from build123d import *

# Parameters (mm, degrees)
BOSS_EXTRUDE1_DEPTH = 80
CUT_EXTRUDE4_DEPTH  = 86.022442091
SKETCH3_W           = 85.02244209
SKETCH3_H           = 14.481412897
CUT_EXTRUDE5_DEPTH  = 61.793248749
SKETCH4_R           = 11.893880873
CUT_EXTRUDE6_DEPTH  = 86.022442091


with BuildPart() as part:
    # Sketch1 → Boss-Extrude1 (new body)
    with BuildSketch(Plane.XY):
        with BuildLine():
            Line((40.088301711, 44.273344197), (40.088301711, -18.282027703))
            ThreePointArc((40.088301711, -18.282027703), (-2.422919334, -60.793248749), (-44.934140379, -18.282027703))
            Line((-44.934140379, -18.282027703), (-44.934140379, 44.273344197))
            Line((-44.934140379, 44.273344197), (-28.193970434, 44.273344197))
            Line((-28.193970434, 44.273344197), (-28.193970434, -18.282027703))
            ThreePointArc((-28.193970434, -18.282027703), (-2.643184728, -43.832813409), (22.907600978, -18.282027703))
            Line((22.907600978, -18.282027703), (22.907600978, 44.273344197))
            Line((22.907600978, 44.273344197), (40.088301711, 44.273344197))
        make_face()
    extrude(amount=-BOSS_EXTRUDE1_DEPTH)

    # Sketch2 → Cut-Extrude4 (cut, through all)
    with BuildSketch(Plane(origin=(40.088301711, 0, 0), x_dir=(0, 0, -1), z_dir=(1, 0, 0))):
        with BuildLine():
            Line((14.481412897, -18.282027703), (14.481412897, 12.995658247))
            ThreePointArc((14.481412897, 12.995658247), (40, 38.51424535), (65.518587103, 12.995658247))
            Line((65.518587103, 12.995658247), (65.518587103, -18.282027703))
            Line((65.518587103, -18.282027703), (80, -18.282027703))
            Line((80, -18.282027703), (80, 44.273344197))
            Line((80, 44.273344197), (0, 44.273344197))
            Line((0, 44.273344197), (0, -18.282027703))
            Line((0, -18.282027703), (14.481412897, -18.282027703))
        make_face()
    extrude(amount=-CUT_EXTRUDE4_DEPTH, mode=Mode.SUBTRACT)

    # Sketch3 → Cut-Extrude5 (cut, through all)
    with BuildSketch(Plane(origin=(0, 0, 0), x_dir=(1, 0, 0), z_dir=(0, 1, 0))):
        with Locations((-2.422919334, 7.240706449)):
            Rectangle(SKETCH3_W, SKETCH3_H)
        with Locations((-2.422919334, 72.759293552)):
            Rectangle(SKETCH3_W, SKETCH3_H)
    extrude(amount=-CUT_EXTRUDE5_DEPTH, mode=Mode.SUBTRACT)

    # Sketch4 → Cut-Extrude6 (cut, through all)
    with BuildSketch(Plane(origin=(40.088301711, 0, 0), x_dir=(0, 0, -1), z_dir=(1, 0, 0))):
        with Locations((40, 12.995658247)):
            Circle(SKETCH4_R)
    extrude(amount=-CUT_EXTRUDE6_DEPTH, mode=Mode.SUBTRACT)


solid = part.part
Check sheet for the modelled part. Datum: model origin and axes. Units: mm. A direction names the side the tool comes from. Give positions to 0.01 mm unless a question says otherwise; leave off trailing zeros. Loops run counter-clockwise (first coordinate to the right, second up) from the corner with the lowest first, then second, coordinate; pieces in that order, holes last. Notation, with made-up numbers: M 15,25.5 L 62,25.5 A5 cw 62,33.5 Z; hole C 8,22 d9. An arc over 180 degrees is marked long. Use a Markdown table: item, result. Add a question column.
Q1. Go/stop test with flat-tipped pins: pin 1 (3 mm diameter, centred on x = -20.5, z = -43, fed in from +Y); pin 2 (10 mm diameter, centred on x = 27.5, z = -55.5, fed in from -Y); pin 3 (1.5 mm diameter, centred on x = -34.5, z = -34, fed in from +Y). Record where each tip stops, or that it passes through.
Q2. Sectioned sample at A-A, the plane y = -14.5. Record the cut outline in (x, z), then the cut area to 3 significant figures.
Q3. Sectioned sample at C-C, the plane y = -41. Record the cut outline in (x, z), then the cut area to 3 significant figures.
Q4. Scan lines: line 1 along X through (y, z) = (-11, -56); line 2 along X through (y, z) = (-22, -52); line 3 along Y through (x, z) = (26, -31). Record each from-to range of solid material in increasing order. Write a range as [from, to].
Q5. Sectioned sample at D-D, the plane z = -24. Record the cut outline in (x, y).
Q6. Mould release check, pull along X, two halves, no side actions. Record for faces 1 (the flat face through (-3, -48, -65.519)), 2 (the cylindrical face through (-3.205, -43.827, -39.643)), 3 (the cylindrical face through (-1.488, -60.783, -39.643)), 4 (the flat face through (-44.934, -3, -40)): pulls with the +X half, pulls with the -X half, needs draft (parallel to the pull), parting line crosses it, or undercut.
Q7. Sectioned sample at B-B, the plane z = -40. Record the cut outline in (x, y).
Q8. Tool access check on faces 5 (the flat face through (22.908, -3, -40)), 6 (the cylindrical face through (-36.45, 38.51, -39.44)). Record the directions out of +Z, -Z, +X, -X, +Y, -Y that give a thin tool (end or side, any length) a straight path to the whole face; none if there is none.
Verdict:
| question | item | result |
|---|---|---|
| 1 | pin 1 | y = -34.96 |
| 1 | pin 2 | y = -52.72 |
| 1 | pin 3 | y = 37.97 |
| 2 | outline | M -44.93,-65.52 L -28.19,-65.52 L -28.19,-14.48 L -44.93,-14.48 Z; M 22.91,-65.52 L 40.09,-65.52 L 40.09,-14.48 L 22.91,-14.48 Z |
| 2 | area | 1,730 mm^2 |
| 3 | outline | M -38.35,-65.52 L -14.34,-65.52 L -14.34,-14.48 L -38.35,-14.48 Z; M 9.05,-65.52 L 33.51,-65.52 L 33.51,-14.48 L 9.05,-14.48 Z |
| 3 | area | 2,470 mm^2 |
| 4 | line 1 | [-44.93, -28.19], [22.91, 40.09] |
| 4 | line 2 | [-44.77, -27.92], [22.64, 39.93] |
| 4 | line 3 | [-49.89, 5.22], [20.77, 36.87] |
| 5 | outline | M -44.93,-18.28 A42.51 ccw 40.09,-18.28 L 40.09,32.88 L 22.91,32.88 L 22.91,-18.28 A25.55 cw -28.19,-18.28 L -28.19,32.88 L -44.93,32.88 Z |
| 6 | face 1 | needs draft |
| 6 | face 2 | undercut |
| 6 | face 3 | parting line crosses it |
| 6 | face 4 | pulls with the -X half |
| 7 | outline | M -44.93,-18.28 A42.51 ccw 40.09,-18.28 L 40.09,1.1 L 22.91,1.1 L 22.91,-18.28 A25.55 cw -28.19,-18.28 L -28.19,1.1 L -44.93,1.1 Z; M -44.93,24.89 L -28.19,24.89 L -28.19,38.51 L -44.93,38.51 Z; M 22.91,24.89 L 40.09,24.89 L 40.09,38.51 L 22.91,38.51 Z |
| 8 | face 5 | +Z, -Z, +Y |
| 8 | face 6 | +X, -X, +Y |
